```python
from build123d import *

# Parameters (mm, degrees)
F0_R     = 1.5
F1_DEPTH = 3
F3_DEPTH = 5


with BuildPart() as f1:
    # F0 (on Right) → F1 (new body)
    with BuildSketch(Plane.YZ):
        Circle(F0_R)
    extrude(amount=F1_DEPTH)

    # F2 (on face) → F3 (join)
    with BuildSketch(Plane.YZ.offset(3)):
        with BuildLine():
            Line((4, -10), (4, 0))
            ThreePointArc((4, 0), (0, 4), (-4, 0))
            Line((-4, 0), (-4, -10))
            Line((-4, -10), (4, -10))
        make_face()
    extrude(amount=F3_DEPTH)


solid = f1.part
```
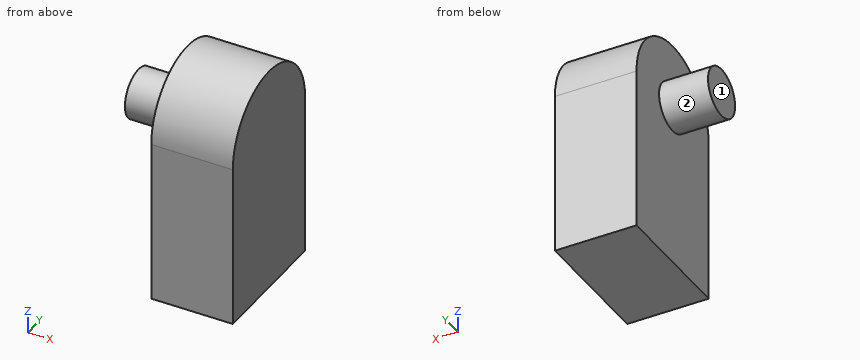
Check sheet for the modelled part. Datum: model origin and axes. Units: mm. Face numbers are marked on the shaded views. A direction names the side the tool comes from. Round coordinates to 2 decimals unless told otherwise and drop trailing zeros. Loops run counter-clockwise (first coordinate to the right, second up) from the corner with the lowest first, then second, coordinate; pieces in that order, holes last. Notation, with made-up numbers: (36, 49.5) - (44, 49.5) arc R27 ccw to (44, 70.5) - close; hole circle Ø1 at (41.25, 33.5). An arc over 180 degrees is marked (long way). Write item = value, one per line. Start each with the question number.
Q1. Depth check by flat-ended pin: P1, Ø1.5, axis at x = 1, z = -6.5, coming from the -Y side; P2, Ø2, axis at x = 1.5, y = -1, coming from the -Z side; P3, Ø2, axis at x = 5.5, y = -1.5, coming from the +Z side. Enter the tip coordinate at first touch or a pass-through.
Q2. Section check C-C (z = -8.5). Record the boundary of the cut face in (x, y), plus the area to 3 significant figures.
Q3. Section check B-B (x = 6.25). Record the boundary of the cut face in (y, z).
Q4. Section check A-A (y = 0). Record the boundary of the cut face in (x, z).
Q5. Access from +Z, -Z, +X, -X, +Y, -Y to the whole of each face (thin tool, end or side, straight path). Record for the marked faces 1 and 2.
Q6. Section check D-D (x = 1). Record the boundary of the cut face in (y, z), plus the area to 3 significant figures.
Q7. Thickness scan on L1, parallel to X at y = 1, z = 2.5; L2, parallel to Z at x = 4, y = 1.75; L3, parallel to Y at x = 5.5, z = 1. Record the ranges inside material, lowest first.
Derived:
q1.P1 = through
q1.P2 = -1.5
q1.P3 = 3.97
q2.outline = (3, -4) - (8, -4) - (8, 4) - (3, 4) - close
q2.area = 40.0 mm^2
q3.outline = (-4, -10) - (4, -10) - (4, 0) arc R4 ccw to (-4, 0) - close
q4.outline = (0, -1.5) - (3, -1.5) - (3, -10) - (8, -10) - (8, 4) - (3, 4) - (3, 1.5) - (0, 1.5) - close
q5.face_1 = +Z, -Z, -X, +Y, -Y
q5.face_2 = -X
q6.outline = circle Ø3 at (0, 0)
q6.area = 7.07 mm^2
q7.L1 = 3 to 8
q7.L2 = -10 to 3.6
q7.L3 = -3.87 to 3.87
